Input: part model. Units: mm. Frame: model coordinates. Round coordinates to 2 decimals unless told otherwise and drop trailing zeros. Write each loop counter-clockwise with the first axis right and the second up, starting at its lowest first coordinate (ties: lowest second). Pieces come first, ordered by that corner, then holes. Notation, with made-up numbers: M 51,78 L 73,78 A21 ccw 73,84 Z; hole C 11,57.25 d1. An arc over 180 degrees is marked long. Use one line per item in the form item = value. Start each with the question number.
```python
from build123d import *

# Parameters (mm, degrees)
SKETCH1_R                        = 30
TANDHJUL_MAINBODY_DEPTH          = 1
SKETCH2_R                        = 15
TANDHJUL_FISKELINIE_DEPTH        = 20
SKETCH3_R                        = 17.5
TANDHJUL_FISKELINIESTOPPER_DEPTH = 1
T_NDER_DEPTH                     = 1
T_NDERPATTERN_COUNT              = 30
SKETCH11_R                       = 17.5
BOSS_EXTRUDE1_DEPTH              = 5
SKETCH12_R                       = 21
BOSS_EXTRUDE2_DEPTH              = 14
FILLET1_R                        = 2
SKETCH13_R                       = 18.5
CUT_EXTRUDE1_DEPTH               = 12
SKETCH14_R                       = 17
CUT_EXTRUDE2_DEPTH               = 2
SKETCH15_R                       = 23.679719335
CUT_EXTRUDE3_DEPTH               = 10
SKETCH18_R                       = 17.5
BOSS_EXTRUDE3_DEPTH              = 2


with BuildPart() as part:
    # Sketch1 → Tandhjul mainBody (new body)
    with BuildSketch(Plane(origin=(0, 0, 0), x_dir=(1, 0, 0), z_dir=(0, 1, 0))):
        Circle(SKETCH1_R)
    extrude(amount=TANDHJUL_MAINBODY_DEPTH)

    # Sketch2 → Tandhjul fiskelinie (add)
    with BuildSketch(Plane(origin=(0, 1, 0), x_dir=(1, 0, 0), z_dir=(0, 1, 0))):
        Circle(SKETCH2_R)
    extrude(amount=TANDHJUL_FISKELINIE_DEPTH)

    # Sketch3 → Tandhjul fiskelinieStopper (add)
    with BuildSketch(Plane(origin=(0, 21, 0), x_dir=(1, 0, 0), z_dir=(0, 1, 0))):
        Circle(SKETCH3_R)
    extrude(amount=TANDHJUL_FISKELINIESTOPPER_DEPTH)

    # Sketch9 → Tænder (add)
    with BuildSketch(Plane(origin=(0, 1, 0), x_dir=(1, 0, 0), z_dir=(0, 1, 0))):
        Polygon((-1.5, 37.197102186), (-5.038144939, 23.992565508), (0, 23.992565508), (5.038144939, 23.992565508), (1.5, 37.197102186), align=None)
    t_nder = extrude(amount=-T_NDER_DEPTH)

    # TænderPattern: Tænder ×30 about axis
    t_nderpattern_axis = Axis((0, 0, 0), (0, 1, 0))
    for i in range(1, T_NDERPATTERN_COUNT):
        add(t_nder.rotate(t_nderpattern_axis, i * 360 / T_NDERPATTERN_COUNT))

    # Sketch11 → Boss-Extrude1 (add)
    with BuildSketch(Plane(origin=(0, 1, 0), x_dir=(1, 0, 0), z_dir=(0, 1, 0))):
        Circle(SKETCH11_R)
    extrude(amount=BOSS_EXTRUDE1_DEPTH)

    # Sketch12 → Boss-Extrude2 (add)
    with BuildSketch(Plane.XZ):
        Circle(SKETCH12_R)
    extrude(amount=BOSS_EXTRUDE2_DEPTH)

    # Fillet1
    fillet1_edges = [part.edges().sort_by_distance(p)[0] for p in [
        (-21, 0, 0),
    ]]
    fillet(fillet1_edges, radius=FILLET1_R)

    # Sketch13 → Cut-Extrude1 (cut)
    with BuildSketch(Plane.XZ.offset(14)):
        Circle(SKETCH13_R)
    extrude(amount=-CUT_EXTRUDE1_DEPTH, mode=Mode.SUBTRACT)

    # Sketch14 → Cut-Extrude2 (cut)
    with BuildSketch(Plane.XZ.offset(2)):
        Circle(SKETCH14_R)
    extrude(amount=-CUT_EXTRUDE2_DEPTH, mode=Mode.SUBTRACT)

    # Sketch15 → Cut-Extrude3 (cut)
    with BuildSketch(Plane(origin=(0, 22, 0), x_dir=(1, 0, 0), z_dir=(0, 1, 0))):
        with Locations((-1.024461649, -1.098868056)):
            Circle(SKETCH15_R)
    extrude(amount=-CUT_EXTRUDE3_DEPTH, mode=Mode.SUBTRACT)

    # Sketch18 → Boss-Extrude3 (add)
    with BuildSketch(Plane(origin=(0, 12, 0), x_dir=(1, 0, 0), z_dir=(0, 1, 0))):
        Circle(SKETCH18_R)
    extrude(amount=BOSS_EXTRUDE3_DEPTH)


solid = part.part
```
Item 1: Cut plane C-C (y = 2). Output: boundary loops of the cut face in (x, z), plus the area to 3 significant figures.
Item 2: Draft query along X for faces 1 (the face through (-13.887, 3.465, 10.648)), 2 (the face through (-2.38, 0.51, 33.92)), 3 (the face through (27.629, 0.507, 24.905)). Return one class per face: +X half, -X half, draft (parallel to the pull), parting line (faces both ways), or undercut.
Item 3: First-contact query: pin 1 (10 mm diameter, centred on x = 4, z = 28.5, fed in from +Y); pin 2 (3 mm diameter, centred on y = 9.5, z = -3.5, fed in from +X); pin 3 (2 mm diameter, centred on x = 2, z = 11.5, fed in from -Y). Flat tips, straight axial feed; report the tip coordinate or a pass-through.
Item 4: Ray query, line 1 (Z direction, x = 0, y = -8); line 2 (Y direction, x = 1, z = -27); line 3 (Y direction, x = 8, z = -5). Return the intervals inside material, ascending. Write a range as from..to.
Item 5: Cut plane D-D (y = 9.25). Output: boundary loops of the cut face in (x, z).
Item 6: Cut plane B-B (y = -6). Output: boundary loops of the cut face in (x, z).
Final values:
q1.outline = C 0,0 d35
q1.area = 962 mm^2
q2.face_1 = parting line
q2.face_2 = undercut
q2.face_3 = +X half
q3.pin_1 = 1
q3.pin_2 = 14.87
q3.pin_3 = 0
q4.line_1 = -21..-18.5, 18.5..21
q4.line_2 = 0..1
q4.line_3 = 0..14
q5.outline = C 0,0 d30
q6.outline = C 0,0 d42; hole C 0,0 d37
